The listing builds one solid part. Answer for the finished solid, in the listing's coordinates (mm). A direction names the side the tool comes from. Coordinates: 2 decimals unless noted, no trailing zeros. Loops run counter-clockwise (first coordinate to the right, second up) from the corner with the lowest first, then second, coordinate; pieces in that order, holes last. Notation, with made-up numbers: (-32.5, -7.5) -> (11.5, -7.5) arc R17 ccw to (11.5, -1.5) -> close; hole circle Ø11 at (38, 6). An arc over 180 degrees is marked (long way). Answer in a Markdown table with one row per item.
```python
from build123d import *

# Parameters (mm, degrees)
F1_DEPTH = 2
F3_DEPTH = 20.5
F5_DEPTH = 10


with BuildPart() as f1:
    # F0 (on Right) → F1 (new body)
    with BuildSketch(Plane.YZ):
        Polygon((10, 0), (0, 0), (0, -2), (12, -2), (12, 20.5), (10, 20.5), align=None)
    extrude(amount=F1_DEPTH)

    # F2 (on face) → F3 (cut)
    with BuildSketch(Plane.XY.offset(20.5)):
        with BuildLine():
            ThreePointArc((0, 11), (0.292893, 11.707107), (1, 12))
            Line((1, 12), (0, 12))
            Line((0, 12), (0, 11))
        make_face()
        with BuildLine():
            ThreePointArc((1, 12), (1.707107, 11.707107), (2, 11))
            Line((2, 11), (2, 12))
            Line((2, 12), (1, 12))
        make_face()
        with BuildLine():
            Line((2, 10), (2, 11))
            ThreePointArc((2, 11), (1.707107, 10.292893), (1, 10))
            Line((1, 10), (2, 10))
        make_face()
        with BuildLine():
            Line((0, 10), (1, 10))
            ThreePointArc((1, 10), (0.292893, 10.292893), (0, 11))
            Line((0, 11), (0, 10))
        make_face()
    extrude(amount=-F3_DEPTH, mode=Mode.SUBTRACT)

    # F4 (on face) → F5 (cut)
    with BuildSketch(Plane.XZ):
        with BuildLine():
            Line((0, -2), (1, -2))
            ThreePointArc((1, -2), (0.292893, -1.707107), (0, -1))
            Line((0, -1), (0, -2))
        make_face()
        with BuildLine():
            Line((2, -2), (2, -1))
            ThreePointArc((2, -1), (1.707107, -1.707107), (1, -2))
            Line((1, -2), (2, -2))
        make_face()
        with BuildLine():
            ThreePointArc((1, 0), (1.707107, -0.292893), (2, -1))
            Line((2, -1), (2, 0))
            Line((2, 0), (1, 0))
        make_face()
        with BuildLine():
            ThreePointArc((0, -1), (0.292893, -0.292893), (1, 0))
            Line((1, 0), (0, 0))
            Line((0, 0), (0, -1))
        make_face()
    extrude(amount=-F5_DEPTH, mode=Mode.SUBTRACT)


solid = f1.part
```
Item 1: A cutting plane is placed at D-D, the plane x = 0.6. Determine the outline of the cut face in (y, z).
Findings below:
| item | result |
|---|---|
| outline | (0, -1.92) -> (10, -1.92) -> (10, -2) -> (12, -2) -> (12, 0) -> (11.92, 0) -> (11.92, 20.5) -> (10.08, 20.5) -> (10.08, 0) -> (10, 0) -> (10, -0.08) -> (0, -0.08) -> close |
Item 2: A cutting plane is placed at A-A, the plane x = 1.6. Determine the outline of the cut face in (y, z).
Findings below:
| item | result |
|---|---|
| outline | (0, -1.8) -> (10, -1.8) -> (10, -2) -> (12, -2) -> (12, 0) -> (11.8, 0) -> (11.8, 20.5) -> (10.2, 20.5) -> (10.2, 0) -> (10, 0) -> (10, -0.2) -> (0, -0.2) -> close |
Item 3: Flat-ended cylindrical pins translate along their axes: pin 1 Ø0.8 at (x, z) = (0.5, -1.5) entering from -Y; pin 2 Ø1 at (x, z) = (1, 4.5) entering from -Y. Find the tip coordinate at first contact, or state that the pin passes through.
Findings below:
| item | result |
|---|---|
| pin 1 | stops at y = 0 |
| pin 2 | stops at y = 10 |
Item 4: Find the intervals of material crossed by probe 1 along Z at (x, y) = (1, 4.5); probe 2 along Y at (x, z) = (1.05, 4.5); probe 3 along Y at (x, z) = (1.45, 6.5), in increasing order.
Findings below:
| item | result |
|---|---|
| probe 1 | z = -2 to 0 |
| probe 2 | y = 10 to 12 |
| probe 3 | y = 10.11 to 11.89 |
Item 5: A cutting plane is placed at C-C, the plane z = 8. Determine the outline of the cut face in (x, y), plus the area to 3 significant figures.
Findings below:
| item | result |
|---|---|
| outline | (0, 11) arc R1 ccw to (1, 10) arc R1 ccw to (2, 11) arc R1 ccw to (1, 12) arc R1 ccw to start |
| area | 3.14 mm2 |
Item 6: A tool of negligible diameter and unlimited length cuts with its end or side. For faces 1 (the face through (1, 11, 20.5)), 2 (the face through (1.79, 11.84, 0)), 3 (the face through (0.16, 10.21, 0)), 4 (the face through (1.79, 10, -0.16)), from which of +Z, -Z, +X, -X, +Y, -Y can it reach the whole face along a straight path? Write none if from no direction.
Findings below:
| item | result |
|---|---|
| face 1 | +Z, +X, -X, +Y, -Y |
| face 2 | +Z, +X, +Y |
| face 3 | +Z, -X, -Y |
| face 4 | +Z, +X, -Y |
